Could you check a few things on this model? Use its own coordinates, in mm. Coordinates: 2 decimals unless noted, no trailing zeros. Loops run counter-clockwise (first coordinate to the right, second up) from the corner with the lowest first, then second, coordinate; pieces in that order, holes last. Notation, with made-up numbers: M 51.5,14.25 L 107.5,14.25 A13 ccw 107.5,32.25 Z; hole C -14,59.25 d2. An arc over 180 degrees is marked long. Return JSON: item names as keys, results as strings. Group by question number.
from build123d import *

# Parameters (mm, degrees)
F1_DEPTH = 7
F2_R     = 2
F3_SIZE  = 1


with BuildPart() as f1:
    # F0 (on Top) → F1 (new body)
    with BuildSketch(Plane.XY):
        with BuildLine():
            ThreePointArc((-12.6158602151, 3.4344862839), (-12.1873110001, 4.7355121779), (-11.625, 5.9845634761))
            ThreePointArc((-11.625, 5.9845634761), (-36.325, 0), (-11.625, -5.9845634761))
            ThreePointArc((-11.625, -5.9845634761), (-12.1873110001, -4.7355121779), (-12.6158602151, -3.4344862839))
            ThreePointArc((-12.6158602151, -3.4344862839), (-34.425, 0), (-12.6158602151, 3.4344862839))
        make_face()
        with BuildLine():
            ThreePointArc((-10.6341397849, 3.4344862839), (0, 11.175), (10.6341397849, 3.4344862839))
            ThreePointArc((10.6341397849, 3.4344862839), (11.0626889999, 4.7355121779), (11.625, 5.9845634761))
            ThreePointArc((11.625, 5.9845634761), (0, 13.075), (-11.625, 5.9845634761))
            ThreePointArc((-11.625, 5.9845634761), (-11.0626889999, 4.7355121779), (-10.6341397849, 3.4344862839))
        make_face()
        with BuildLine():
            ThreePointArc((36.325, 0), (26.3288593667, 12.7073305615), (11.625, 5.9845634761))
            ThreePointArc((11.625, 5.9845634761), (12.1873110001, 4.7355121779), (12.6158602151, 3.4344862839))
            ThreePointArc((12.6158602151, 3.4344862839), (24.9884062965, 11.0389568596), (34.425, 0))
            ThreePointArc((34.425, 0), (24.9884062965, -11.0389568596), (12.6158602151, -3.4344862839))
            ThreePointArc((12.6158602151, -3.4344862839), (12.1873110001, -4.7355121779), (11.625, -5.9845634761))
            ThreePointArc((11.625, -5.9845634761), (26.3288593667, -12.7073305615), (36.325, 0))
        make_face()
        with BuildLine():
            ThreePointArc((11.625, -5.9845634761), (11.0626889999, -4.7355121779), (10.6341397849, -3.4344862839))
            ThreePointArc((10.6341397849, -3.4344862839), (0, -11.175), (-10.6341397849, -3.4344862839))
            ThreePointArc((-10.6341397849, -3.4344862839), (-11.0626889999, -4.7355121779), (-11.625, -5.9845634761))
            ThreePointArc((-11.625, -5.9845634761), (0, -13.075), (11.625, -5.9845634761))
        make_face()
        with BuildLine():
            ThreePointArc((10.6341397849, 3.4344862839), (11.0389568596, 1.7384062965), (11.175, 0))
            ThreePointArc((11.175, 0), (11.0389568596, -1.7384062965), (10.6341397849, -3.4344862839))
            ThreePointArc((10.6341397849, -3.4344862839), (11.0626889999, -4.7355121779), (11.625, -5.9845634761))
            ThreePointArc((11.625, -5.9845634761), (12.1873110001, -4.7355121779), (12.6158602151, -3.4344862839))
            ThreePointArc((12.6158602151, -3.4344862839), (12.075, 0), (12.6158602151, 3.4344862839))
            ThreePointArc((12.6158602151, 3.4344862839), (12.1873110001, 4.7355121779), (11.625, 5.9845634761))
            ThreePointArc((11.625, 5.9845634761), (11.0626889999, 4.7355121779), (10.6341397849, 3.4344862839))
        make_face()
        with BuildLine():
            ThreePointArc((-10.6341397849, -3.4344862839), (-11.175, 0), (-10.6341397849, 3.4344862839))
            ThreePointArc((-10.6341397849, 3.4344862839), (-11.0626889999, 4.7355121779), (-11.625, 5.9845634761))
            ThreePointArc((-11.625, 5.9845634761), (-12.1873110001, 4.7355121779), (-12.6158602151, 3.4344862839))
            ThreePointArc((-12.6158602151, 3.4344862839), (-12.2110431404, 1.7384062965), (-12.075, 0))
            ThreePointArc((-12.075, 0), (-12.2110431404, -1.7384062965), (-12.6158602151, -3.4344862839))
            ThreePointArc((-12.6158602151, -3.4344862839), (-12.1873110001, -4.7355121779), (-11.625, -5.9845634761))
            ThreePointArc((-11.625, -5.9845634761), (-11.0626889999, -4.7355121779), (-10.6341397849, -3.4344862839))
        make_face()
    extrude(amount=F1_DEPTH)

    # F2
    f2_edges = [f1.edges().sort_by_distance(p)[0] for p in [
        (-11.625, -5.984563, 3.5),
        (11.625, -5.984563, 3.5),
        (-11.625, 5.984563, 3.5),
        (11.625, 5.984563, 3.5),
    ]]
    fillet(f2_edges, radius=F2_R)

    # F3
    f3_edges = [f1.edges().sort_by_distance(p)[0] for p in [
        (0, -13.075, 7),
        (-36.325, 0, 0),
    ]]
    chamfer(f3_edges, length=F3_SIZE)


solid = f1.part
(1) Imagine slicing it at B-B, the plane z = 3.5. Count the separate pieces of the cut face and the enclosed holes in it, then the cut area to 4 significant figures.
(2) We'd pull the mould along X, two halves only. Please class faces 1 (the face through (10.3, 5.4, 0)), 2 (the face through (-0.151, -12.248, 6.826)): +X half, -X half, draft (parallel to the pull), parting line (faces both ways), or undercut.
(3) Will these pins go through, and if not, where does the flat tip stop? P1, Ø13.5, axis at x = -23.25, y = 0, coming from the -Z side; P2, Ø4, axis at y = -7.5, z = 6, coming from the +X side; P3, Ø1.5, axis at x = -18, z = 4.5, coming from the -Y side; P4, Ø1, axis at x = -1, z = 2, coming from the +Y side.
(4) Imagine slicing it at A-A, the plane x = -23.25. Write out the boundary of the cut face in (y, z) (3 decimals), then the cut area to 3 significant figures.
(5) If I drill on L1, parallel to Y at x = -23.25, z = 3 (3 decimals); L2, parallel to X at y = 1, z = 3.25; L3, parallel to X at y = 8.75, z = 4.5, over which ranges is the centre line in solid material (lowest first)? Write a range as [from, to].
Checks:
{
 "1": {"separate pieces": "1", "enclosed holes": "3", "area": "394.5 mm²"},
 "2": {"face 1": "draft", "face 2": "undercut"},
 "3": {"P1": "through", "P2": "x = 35.11", "P3": "y = -12.28", "P4": "y = 13.07"},
 "4": {"outline": "M -13.075,1 L -12.075,0 L -11.175,0 L -11.175,7 L -12.075,7 L -13.075,6 Z; M 11.175,0 L 12.075,0 L 13.075,1 L 13.075,6 L 12.075,7 L 11.175,7 Z", "area": "24.6 mm²"},
 "5": {"L1": "[-13.075, -11.175], [11.175, 13.075]", "L2": "[-36.29, -34.38], [-12.12, -11.13], [11.13, 12.12], [34.38, 36.29]", "L3": "[-32.97, -30.2], [-16.3, -13.53], [-9.72, -6.95], [6.95, 9.72], [13.53, 16.3], [30.2, 32.97]"}
}
